```python
from build123d import *

# Parameters (mm, degrees)
F1_DEPTH = 35
F2_DEPTH = 5
F3_DEPTH = 5
F4_DEPTH = 8


with BuildPart() as f1:
    # F0 (on Top) → F1 (new body)
    with BuildSketch(Plane.XY):
        Polygon((-4.5421427263, -18.7091076313), (-7.1265365105, -23.1058005667), (-0.2120626165, -27.170156121), (7.0488793967, -23.0532723663), (4.5334285141, -18.6167752281), (22.1390458625, -8.6345608102), (20.9306429875, -6.5033023811), (-0.1440209293, -18.4524325843), (-21.0296031968, -6.1758033577), (-22.271125701, -8.28794016), align=None)
        Polygon((-24.8555194852, -12.6846330954), (-26.0970419893, -14.7967698977), (-0.2341423693, -29.9990862753), (12.8143786254, -22.6007013264), (25.8628996201, -15.2023163775), (24.6544967451, -13.0710579484), (7.0488793967, -23.0532723663), (-0.2120626165, -27.170156121), (-7.1265365105, -23.1058005667), align=None)
    extrude(amount=F1_DEPTH)

    # F0 (on Top) → F2 (join)
    with BuildSketch(Plane.XY):
        Polygon((-22.271125701, -8.28794016), (-24.8555194852, -12.6846330954), (-7.1265365105, -23.1058005667), (-4.5421427263, -18.7091076313), align=None)
        Polygon((7.0488793967, -23.0532723663), (24.6544967451, -13.0710579484), (22.1390458625, -8.6345608102), (4.5334285141, -18.6167752281), align=None)
    extrude(amount=F2_DEPTH)

    # F0 (on Top) → F3 (join)
    with BuildSketch(Plane.XY):
        with BuildLine():
            Line((12.8143786254, -22.6007013264), (-0.2341423693, -29.9990862753))
            ThreePointArc((-0.2341423693, -29.9990862753), (8.7789969459, -35.8134839164), (19.3797362449, -34.1800132069))
            Line((19.3797362449, -34.1800132069), (18.0699600882, -31.8699628652))
            ThreePointArc((18.0699600882, -31.8699628652), (12.6174518365, -30.3632599197), (14.1241547821, -24.9107516681))
            Line((14.1241547821, -24.9107516681), (12.8143786254, -22.6007013264))
        make_face()
        with BuildLine():
            Line((25.8628996201, -15.2023163775), (12.8143786254, -22.6007013264))
            Line((12.8143786254, -22.6007013264), (14.1241547821, -24.9107516681))
            ThreePointArc((14.1241547821, -24.9107516681), (18.1105605252, -24.9340868337), (20.0970574351, -28.3903572667))
            ThreePointArc((20.0970574351, -28.3903572667), (19.5533278681, -30.4038603568), (18.0699600882, -31.8699628652))
            Line((18.0699600882, -31.8699628652), (19.3797362449, -34.1800132069))
            ThreePointArc((19.3797362449, -34.1800132069), (26.2244652335, -25.9220724639), (25.8628996201, -15.2023163775))
        make_face()
    extrude(amount=F3_DEPTH)

    # F0 (on Top) → F4 (join)
    with BuildSketch(Plane.XY):
        with BuildLine():
            Line((15.3572189402, -27.0855051672), (14.1241547821, -24.9107516681))
            ThreePointArc((14.1241547821, -24.9107516681), (12.6174518365, -30.3632599197), (18.0699600882, -31.8699628652))
            Line((18.0699600882, -31.8699628652), (16.83689593, -29.6952093661))
            ThreePointArc((16.83689593, -29.6952093661), (14.7922053357, -29.1301957615), (15.3572189402, -27.0855051672))
        make_face()
        with BuildLine():
            ThreePointArc((20.0970574351, -28.3903572667), (18.1105605252, -24.9340868337), (14.1241547821, -24.9107516681))
            Line((14.1241547821, -24.9107516681), (15.3572189402, -27.0855051672))
            ThreePointArc((15.3572189402, -27.0855051672), (16.8521210939, -27.0942558543), (17.5970574351, -28.3903572667))
            ThreePointArc((17.5970574351, -28.3903572667), (17.3931588475, -29.1454209255), (16.83689593, -29.6952093661))
            Line((16.83689593, -29.6952093661), (18.0699600882, -31.8699628652))
            ThreePointArc((18.0699600882, -31.8699628652), (19.5533278681, -30.4038603568), (20.0970574351, -28.3903572667))
        make_face()
    extrude(amount=F4_DEPTH)


solid = f1.part
```
Here's how the part is built. I have some questions about the finished solid (model axes, mm). A direction names the side the tool comes from. Coordinates: 2 decimals unless noted, no trailing zeros. Order: outer loops, then holes, each group sorted by start corner. A loop starts at its lowest first (then second) coordinate and runs counter-clockwise, first axis right, second up. Notation, with made-up numbers: M 36,46.25 L 81,46.25 A24 cw 81,62.25 Z; hole C 10.25,-38 d5. An arc over 180 degrees is marked long. Answer as a JSON object with one key per item and string values. Group by question number.
(1) If we mould it in two halves opening along Y, with no side actions, what happens to faces 6 (the face through (10.541, -12.394, 17.255)), 7 (the face through (-15, -16, 5)), 8 (the face through (13.213, -13.696, 19.79)), 9 (the face through (6, -21, 0))? For each: released by +Y, released by -Y, zero draft, split by the parting line, or undercut.
(2) Suppose I cut it at D-D, the plane x = 10. Please give me the cut outline in (y, z).
(3) Suppose I cut it at A-A, the plane x = 16. Please give me the cut outline in (y, z).
(4) Suppose I cut it at B-B, the plane z = 17. Please give me the cut outline in (x, y), then the cut area to 3 significant figures.
(5) I need wall thicknesses on probe 1 along X at (y, z) = (-15, 18.5); probe 2 along Z at (x, y) = (7.5, -32); probe 3 along X at (y, z) = (-18, 12.5). Which ranges of each line are inside material? Lowest first, please.
(6) Which directions (+Z, -Z, +X, -X, +Y, -Y) give clear straight access to the entire face, cutting with the end or side of a thin tool? Please do faces 1 (the face through (2, -19, 35)), 2 (the face through (16, -30.1, 8)), 3 (the face through (15.975, -17.992, 19.79)), 4 (the face through (-13.35, -22.29, 17.26)), 5 (the face through (-10.44, -12.4, 17.26)).
(7) Suppose I cut it at C-C, the plane y = -22.25. Please give me the cut outline in (x, z).
(8) For pin 1 (3 mm diameter, centred on x = 1.5, z = 30, fed in from +Y); pin 2 (1.5 mm diameter, centred on x = 5, y = -31.5, fed in from +Z); pin 3 (11.5 mm diameter, centred on x = 18.5, y = -14.5, fed in from +Z); pin 4 (1.5 mm diameter, centred on y = -30, z = 30.5, fed in from -X), each with a flat end and sliding along its axis, tell me the tip position at first contact or that it passes through.
Values found:
{
 "1": {"face 6": "released by +Y", "face 7": "undercut", "face 8": "undercut", "face 9": "zero draft"},
 "2": {"outline": "M -36.02,0 L -12.7,0 L -12.7,35 L -15.52,35 L -15.52,5 L -21.38,5 L -21.38,35 L -24.2,35 L -24.2,5 L -36.02,5 Z"},
 "3": {"outline": "M -35.59,0 L -29.89,0 L -29.89,8 L -32.39,8 L -32.39,5 L -35.59,5 Z; M -26.89,0 L -9.3,0 L -9.3,35 L -12.12,35 L -12.12,5 L -17.98,5 L -17.98,35 L -20.79,35 L -20.79,5 L -24.39,5 L -24.39,8 L -26.89,8 Z"},
 "4": {"outline": "M -26.1,-14.8 L -0.23,-30 L 25.86,-15.2 L 24.65,-13.07 L 7.05,-23.05 L 4.53,-18.62 L 22.14,-8.63 L 20.93,-6.5 L -0.14,-18.45 L -21.03,-6.18 L -22.27,-8.29 L -4.54,-18.71 L -7.13,-23.11 L -24.86,-12.68 Z", "area": "334 mm^2"},
 "5": {"probe 1": "x = -25.75 to -20.92, -10.85 to -6.02, 5.95 to 10.91, 21.25 to 25.75", "probe 2": "z = 0 to 5", "probe 3": "x = -20.65 to -15.81, -5.75 to -0.91, 0.65 to 5.62, 15.96 to 20.93"},
 "6": {"face 1": "+Z, +X, -X, +Y, -Y", "face 2": "+Z, +X, -Y", "face 3": "+Z", "face 4": "+Z, -Z, -X, -Y", "face 5": "+Z, -Z, +Y"},
 "7": {"outline": "M -13.42,0 L 26.99,0 L 26.99,5 L 13.43,5 L 13.43,35 L 8.47,35 L 8.47,5 L 6.59,5 L 6.59,35 L -6.62,35 L -6.62,5 L -8.58,5 L -8.58,35 L -13.42,35 Z"},
 "8": {"pin 1": "stops at y = -16.67", "pin 2": "stops at z = 5", "pin 3": "stops at z = 35", "pin 4": "stops at x = -1.51"}
}
